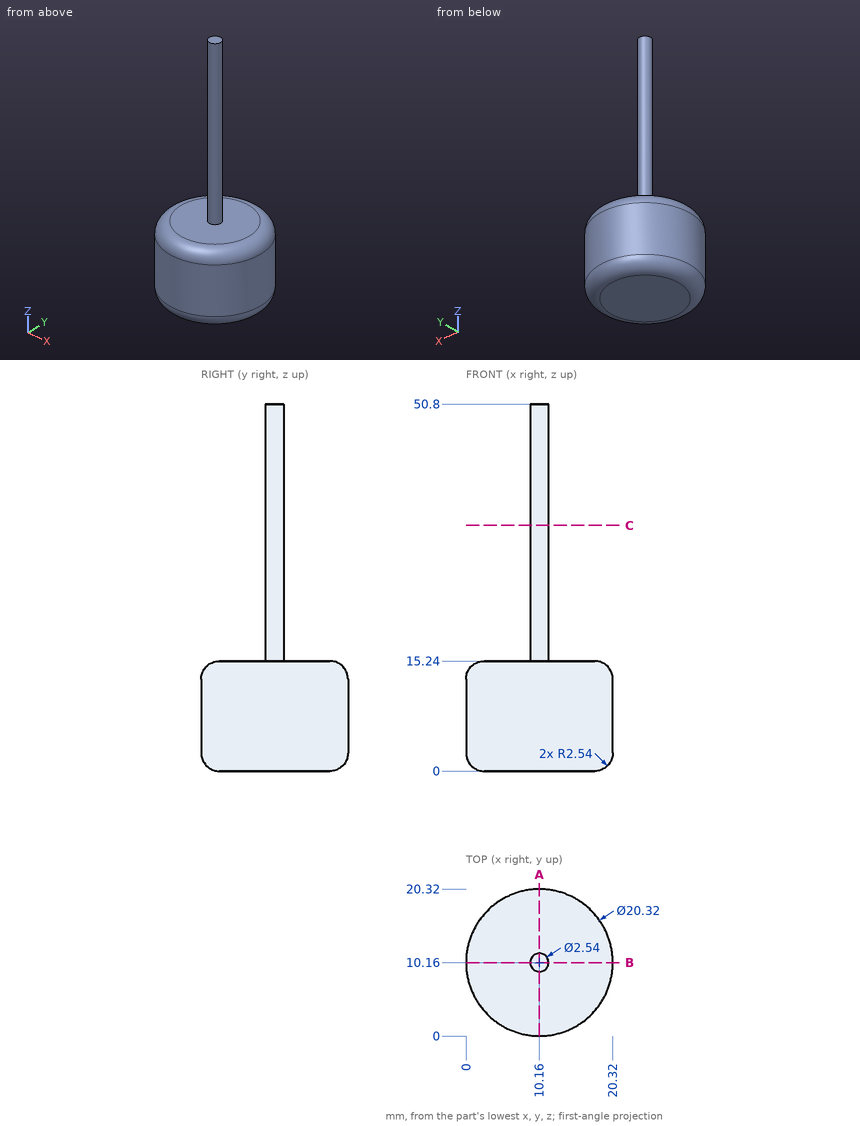
Answer from the drawing. Dimensions are ordinates in mm from the lowest x, y and z of the part. Give positions to 0.01 mm unless a question says otherwise; leave off trailing zeros. Order: outer loops, then holes, each group sorted by start corner. A loop starts at its lowest first (then second) coordinate and runs counter-clockwise, first axis right, second up. Notation, with made-up numbers: (26.5, 0.25) - (43.5, 0.25) arc R28 ccw to (43.5, 37.25) - close; hole circle Ø9 at (87, 46.25). An arc over 180 degrees is marked (long way). One line per item, written item: value. Start each with the question number.
1) Given pin 1 Ø4 at (x, z) = (10, 41.5) entering from +Y; pin 2 Ø5 at (y, z) = (13.5, 15.5) entering from -X; pin 3 Ø5 at (x, z) = (17, 16) entering from -Y, each flat-ended and moving along its own axis, determine where each tip first touches the part or whether it passes through.
2) A cutting plane is placed at A-A on x = 10.16. Give the vertices of the cut face in (y, z), then the cut area to 3 significant figures.
3) A cutting plane is placed at C-C on z = 34. Give the vertices of the cut face in (x, y).
4) Find the intervals of material crossed by L1, parallel to Z at x = 17.5, y = 10.5; L2, parallel to X at y = 8.5, z = 4; L3, parallel to X at y = 3, z = 3, in increasing order.
Answer sheet:
1. pin 1: stops at y = 11.43
1. pin 2: stops at x = 0.3
1. pin 3: stops at y = 1.93
2. outline: (0, 2.54) arc R2.54 ccw to (2.54, 0) - (17.78, 0) arc R2.54 ccw to (20.32, 2.54) - (20.32, 12.7) arc R2.54 ccw to (17.78, 15.24) - (11.43, 15.24) - (11.43, 50.8) - (8.89, 50.8) - (8.89, 15.24) - (2.54, 15.24) arc R2.54 ccw to (0, 12.7) - close
2. area: 394 mm2
3. outline: circle Ø2.54 at (10.16, 10.16)
4. L1: z = 0 to 15.24
4. L2: x = 0.14 to 20.18
4. L3: x = 2.95 to 17.37
